Could you check a few things on this model? Use its own coordinates, in mm. A direction names the side the tool comes from. Coordinates: 2 decimals unless noted, no trailing zeros. Write each loop counter-clockwise with the first axis right and the second up, starting at its lowest first coordinate (ties: lowest second). Pieces come first, ordered by that corner, then holes. Notation, with made-up numbers: (11.25, -35.75) - (55.25, -35.75) arc R11 ccw to (55.25, -17.75) - close; hole circle Ø7 at (80, 40). An arc over 180 degrees is marked (long way). Answer as a JSON object with one key per item and string values. Group by question number.
1) Will these pins go through, and if not, where does the flat tip stop? pin 1 Ø3.5 at (y, z) = (4.5, 2) entering from -X; pin 2 Ø2 at (x, z) = (9.5, 1.5) entering from +Y; pin 3 Ø1.2 at (x, z) = (0, 0) entering from +Y.
2) We'd pull the mould along X, two halves only. Please class faces 1 (the flat face through (16, -14.6, -4)), 2 (the flat face through (-4.505, -15, -5)), 3 (the flat face through (16.62, -8, 0)), 4 (the flat face through (16, -15, 3.55)): released by +X, released by -X, zero draft, split by the parting line, or undercut.
3) If we section it at D-D (z = 0): State how many separate pieces and enclosed holes the cut face has, plus the area to 3 significant figures.
4) If we section it at A-A (y = 2.5): Write out the boundary of the cut face in (x, z) (3 decimals), plus the area to 3 significant figures.
5) If we section it at B-B (x = 0): Write out the boundary of the cut face in (y, z) (3 decimals).
6) If we section it at C-C (y = 11.5): Write out the boundary of the cut face in (x, z) (3 decimals).
7) On a 3-axis mill with a long thin cutter (end or side, diameter ignored), from which of +Z, -Z, +X, -X, +Y, -Y can I reach the whole of each face in a straight line? I mean faces 5 (the flat face through (-5.3, -14.6, -4)), 6 (the cylindrical face through (18, 0.9, 0.1)), 7 (the flat face through (0, 10.5, 0)). Say none if no direction works.
8) Please list where these lines run through material, in increasing order: line 1 along X through (y, z) = (0.6, 0) (3 decimals); line 2 along Z through (x, y) = (-2, 8.25); line 3 along X through (y, z) = (3, -2.25).
```python
from build123d import *

# Parameters (mm, degrees)
BOSS_EXTRUDE1_DEPTH = 6.125
BOSS_EXTRUDE2_DEPTH = 3.8
BOSS_EXTRUDE3_DEPTH = 0.7
SKETCH4_R           = 1
CUT_EXTRUDE1_DEPTH  = 27.766257209
SKETCH5_R           = 0.975
CUT_EXTRUDE2_DEPTH  = 1
BOSS_EXTRUDE6_DEPTH = 0.6
SKETCH9_W           = 1.425
SKETCH9_H           = 3.2
FILLET1_R           = 0.3
FILLET2_R           = 2
FILLET3_R           = 0.5


with BuildPart() as part:
    # Sketch1 → Boss-Extrude1 (new, symmetric)
    with BuildSketch(Plane.XY):
        Polygon((-7.13, 6), (11.92, 6), (16.62, 5.1), (16.62, 1.85), (20.87, 1.85), (20.87, 0), (16.62, 0), (16.62, -15.6), (-7.13, -15.6), (-7.13, 0), (-11.38, 0), (-11.38, 1.85), (-7.13, 1.85), align=None)
    extrude(amount=BOSS_EXTRUDE1_DEPTH, both=True)

    # Sketch2 → Boss-Extrude2 (add)
    with BuildSketch(Plane(origin=(0, 6, 0), x_dir=(1, 0, 0), z_dir=(0, 1, 0))):
        with BuildLine():
            Line((5.251487884, -2.85), (6.125, -2.85))
            ThreePointArc((6.125, -2.85), (8.975, 0), (6.125, 2.85))
            Line((6.125, 2.85), (5.251487884, 2.85))
            ThreePointArc((5.251487884, 2.85), (-5.975, 0), (5.251487884, -2.85))
        make_face()
    extrude(amount=BOSS_EXTRUDE2_DEPTH)

    # Sketch3 → Boss-Extrude3 (add)
    with BuildSketch(Plane(origin=(0, 9.8, 0), x_dir=(1, 0, 0), z_dir=(0, 1, 0))):
        with BuildLine():
            Line((4.498263554, -1.675), (6.125, -1.675))
            ThreePointArc((6.125, -1.675), (7.8, 0), (6.125, 1.675))
            Line((6.125, 1.675), (4.498263554, 1.675))
            ThreePointArc((4.498263554, 1.675), (-4.8, 0), (4.498263554, -1.675))
        make_face()
    extrude(amount=BOSS_EXTRUDE3_DEPTH)

    # Sketch4 → Cut-Extrude1 (cut, through all)
    with BuildSketch(Plane(origin=(0, 0, 0), x_dir=(1, 0, 0), z_dir=(0, 1, 0))):
        with Locations(Location((-9.505, 3.5, 0), (0, 0, 90))):
            Circle(SKETCH4_R)
        with Locations(Location((-9.505, -3.5, 0), (0, 0, 90))):
            Circle(SKETCH4_R)
        with Locations(Location((18.995, 3.5, 0), (0, 0, 90))):
            Circle(SKETCH4_R)
        with Locations(Location((18.995, -3.5, 0), (0, 0, 90))):
            Circle(SKETCH4_R)
        with Locations(Location((18.995, 0, 0), (0, 0, 90))):
            Circle(SKETCH4_R)
        with Locations(Location((-9.505, 0, 0), (0, 0, 90))):
            Circle(SKETCH4_R)
    extrude(amount=CUT_EXTRUDE1_DEPTH, mode=Mode.SUBTRACT)

    # Sketch5 → Cut-Extrude2 (cut)
    # profile 1 of 4: a face of its own
    with BuildSketch(Plane.XZ.offset(15.6)):
        with BuildLine():
            Line((16.62, 6.125), (13.995, 6.125))
            Line((13.995, 6.125), (13.995, 4.85))
            ThreePointArc((13.995, 4.85), (14.375761184, 3.930761184), (15.295, 3.55))
            Line((15.295, 3.55), (16.62, 3.55))
            Line((16.62, 3.55), (16.62, 6.125))
        make_face()
        with Locations(Location((15.395, 4.95, 0), (0, 0, 270))):
            Circle(SKETCH5_R, mode=Mode.SUBTRACT)
    # profile 2 of 4: a face of its own
    with BuildSketch(Plane.XZ.offset(15.6)):
        with BuildLine():
            Line((16.62, -6.125), (13.995, -6.125))
            Line((13.995, -6.125), (13.995, -4.85))
            ThreePointArc((13.995, -4.85), (14.375761184, -3.930761184), (15.295, -3.55))
            Line((15.295, -3.55), (16.62, -3.55))
            Line((16.62, -3.55), (16.62, -6.125))
        make_face()
        with Locations(Location((15.395, -4.95, 0), (0, 0, 270))):
            Circle(SKETCH5_R, mode=Mode.SUBTRACT)
    # profile 3 of 4: a face of its own
    with BuildSketch(Plane.XZ.offset(15.6)):
        with BuildLine():
            Line((-7.13, 6.125), (-4.505, 6.125))
            Line((-4.505, 6.125), (-4.505, 4.85))
            ThreePointArc((-4.505, 4.85), (-4.885761184, 3.930761184), (-5.805, 3.55))
            Line((-5.805, 3.55), (-7.13, 3.55))
            Line((-7.13, 3.55), (-7.13, 6.125))
        make_face()
        with Locations(Location((-5.905, 4.95, 0), (0, 0, 270))):
            Circle(SKETCH5_R, mode=Mode.SUBTRACT)
    # profile 4 of 4: a face of its own
    with BuildSketch(Plane.XZ.offset(15.6)):
        with BuildLine():
            Line((-7.13, -6.125), (-4.505, -6.125))
            Line((-4.505, -6.125), (-4.505, -4.85))
            ThreePointArc((-4.505, -4.85), (-4.885761184, -3.930761184), (-5.805, -3.55))
            Line((-5.805, -3.55), (-7.13, -3.55))
            Line((-7.13, -3.55), (-7.13, -6.125))
        make_face()
        with Locations(Location((-5.905, -4.95, 0), (0, 0, 270))):
            Circle(SKETCH5_R, mode=Mode.SUBTRACT)
    extrude(amount=-CUT_EXTRUDE2_DEPTH, mode=Mode.SUBTRACT)

    # Sketch8 → Boss-Extrude6 (add, symmetric)
    with BuildSketch(Plane.XY):
        Polygon((11.92, 6), (7.8, 6.78893617), (7.8, 6), align=None)
    extrude(amount=BOSS_EXTRUDE6_DEPTH, both=True)

    # Sketch9 → Revolve1 (revolve)
    with BuildSketch(Plane.XY, mode=Mode.PRIVATE) as revolve1_sk:
        with Locations((1.7125, 12.1)):
            Rectangle(SKETCH9_W, SKETCH9_H)
    revolve(revolve1_sk.sketch.rotate(Axis((0, 55, 0), (0, -1, 0)), 90), axis=Axis((0, 55, 0), (0, -1, 0)))

    # Fillet1
    fillet1_edges = [part.edges().sort_by_distance(p)[0] for p in [
        (15.395, -15.6, -3.975),
        (-5.905, -15.6, 5.925),
        (-5.905, -15.6, -3.975),
        (15.395, -15.6, 5.925),
    ]]
    fillet(fillet1_edges, radius=FILLET1_R)

    # Fillet2
    fillet2_edges = [part.edges().sort_by_distance(p)[0] for p in [
        (-11.38, 0.925, 6.125),
        (20.87, 0.925, -6.125),
        (-11.38, 0.925, -6.125),
        (20.87, 0.925, 6.125),
    ]]
    fillet(fillet2_edges, radius=FILLET2_R)

    # Fillet3
    fillet3_edges = [part.edges().sort_by_distance(p)[0] for p in [
        (16.62, -7.3, -6.125),
        (16.62, 3.475, -6.125),
        (-7.13, -7.3, -6.125),
        (-7.13, -7.3, 6.125),
        (-7.13, 3.925, -6.125),
        (16.62, 3.475, 6.125),
        (-7.13, 3.925, 6.125),
        (16.62, -7.3, 6.125),
    ]]
    fillet(fillet3_edges, radius=FILLET3_R)


solid = part.part
```
Here are the results:
{
 "1": {"pin 1": "stops at x = -7.13", "pin 2": "stops at y = 9.8", "pin 3": "stops at y = 10.5"},
 "2": {"face 1": "undercut", "face 2": "undercut", "face 3": "released by +X", "face 4": "zero draft"},
 "3": {"separate pieces": "3", "enclosed holes": "0", "area": "595 mm²"},
 "4": {"outline": "(-7.13, -5.625) arc R0.5 ccw to (-6.63, -6.125) - (16.12, -6.125) arc R0.5 ccw to (16.62, -5.625) - (16.62, 5.625) arc R0.5 ccw to (16.12, 6.125) - (-6.63, 6.125) arc R0.5 ccw to (-7.13, 5.625) - close", "area": "291 mm²"},
 "5": {"outline": "(-15.6, -6.125) - (6, -6.125) - (6, -5.975) - (9.8, -5.975) - (9.8, -4.8) - (10.5, -4.8) - (10.5, -2.425) - (13.7, -2.425) - (13.7, -1) - (10.5, -1) - (10.5, 1) - (13.7, 1) - (13.7, 2.425) - (10.5, 2.425) - (10.5, 4.8) - (9.8, 4.8) - (9.8, 5.975) - (6, 5.975) - (6, 6.125) - (-15.6, 6.125) - close"},
 "6": {"outline": "circle Ø4.85 at (0, 0); hole circle Ø2 at (0, 0)"},
 "7": {"face 5": "-Y", "face 6": "+Y, -Y", "face 7": "+Y"},
 "8": {"line 1": "x = -11.38 to -10.505, -8.505 to 17.995, 19.995 to 20.87", "line 2": "z = -5.63 to 5.63", "line 3": "x = -7.13 to 16.62"}
}
